from build123d import *

# Parameters (mm, degrees)
SKETCH1_R           = 1
BOSS_EXTRUDE1_DEPTH = 3
SKETCH2_W           = 72
SKETCH2_H           = 3
BOSS_EXTRUDE2_DEPTH = 2
SKETCH3_R           = 0.5
CUT_EXTRUDE6_DEPTH  = 1


with BuildPart() as part:
    # Sketch1 → Boss-Extrude1 (new body)
    with BuildSketch(Plane(origin=(0, 0, 0), x_dir=(1, 0, 0), z_dir=(0, 1, 0))):
        with Locations(Location((0, 0, 0), (0, 0, 270))):
            Circle(SKETCH1_R)
    extrude(amount=BOSS_EXTRUDE1_DEPTH)

    # Sketch2 → Boss-Extrude2 (add)
    with BuildSketch(Plane(origin=(0, 3, 0), x_dir=(1, 0, 0), z_dir=(0, 1, 0))):
        with Locations((-35, 0)):
            Rectangle(SKETCH2_W, SKETCH2_H)
    extrude(amount=BOSS_EXTRUDE2_DEPTH)

    # Sketch3 → Cut-Extrude6 (cut)
    with BuildSketch(Plane.XZ.offset(-3)):
        with Locations(Location((-70, 0, 0), (0, 0, 270))):
            Circle(SKETCH3_R)
    extrude(amount=-CUT_EXTRUDE6_DEPTH, mode=Mode.SUBTRACT)


solid = part.part
For this review, take the finished solid that the model builds, in its own axes (mm). A direction names the side the tool comes from. Give positions to 0.01 mm unless a question says otherwise; leave off trailing zeros. Order: outer loops, then holes, each group sorted by start corner. A loop starts at its lowest first (then second) coordinate and runs counter-clockwise, first axis right, second up. Notation, with made-up numbers: (26, 44.5) - (67, 44.5) arc R31 cw to (67, 73.5) - close; hole circle Ø2 at (56, 37). An arc over 180 degrees is marked (long way). Answer as a JSON object with one key per item and string values. Group by question number.
Item 1: Machinability: for faces 1 (the flat face through (0, 0, 0)), 2 (the cylindrical face through (-1, 1, 0)), which of the approach directions +Z, -Z, +X, -X, +Y, -Y give a long, thin tool a straight path to every point of the face, cutting with its end or side? Answer none if there is none.
Item 2: Take a section at B-B on y = 2. Give the boundary of the cut face in (x, z).
Item 3: Take a section at C-C on x = -46.5. Give the boundary of the cut face in (y, z).
Item 4: Take a section at A-A on x = 0. Give the boundary of the cut face in (y, z), and give its area (3 significant figures).
Item 5: Wall thickness on line 1 along X through (y, z) = (3.6, 0); line 2 along Z through (x, y) = (-70, 3.65); line 3 along Y through (x, z) = (-8, -1.05): over which ranges is each line inside the solid? List them lowest first.
Item 6: Clearance check with flat-ended pins moving along their axes: pin 1 Ø3 at (x, y) = (-9.5, 2.5) entering from -Z; pin 2 Ø0.9 at (x, z) = (-23.5, 0.5) entering from -Y; pin 3 Ø1.5 at (y, z) = (2, -1) entering from +X. State where each tip first meets the part, or that it passes through.
Reported:
{
 "1": {"face 1": "+Z, -Z, +X, -X, -Y", "face 2": "-Y"},
 "2": {"outline": "circle Ø2 at (0, 0)"},
 "3": {"outline": "(3, -1.5) - (5, -1.5) - (5, 1.5) - (3, 1.5) - close"},
 "4": {"outline": "(0, -1) - (3, -1) - (3, -1.5) - (5, -1.5) - (5, 1.5) - (3, 1.5) - (3, 1) - (0, 1) - close", "area": "12.0 mm^2"},
 "5": {"line 1": "-71 to -70.5, -69.5 to 1", "line 2": "-1.5 to -0.5, 0.5 to 1.5", "line 3": "3 to 5"},
 "6": {"pin 1": "z = -1.5", "pin 2": "y = 3", "pin 3": "x = 0.97"}
}
